Read the model definition and answer for the solid it produces. Units are mm, in the model's axes. Give positions to 0.01 mm unless a question says otherwise; leave off trailing zeros. Loops run counter-clockwise (first coordinate to the right, second up) from the corner with the lowest first, then second, coordinate; pieces in that order, holes last. Notation, with made-up numbers: (79.5, 62.5) - (123.5, 62.5) arc R19 cw to (123.5, 74.5) - close; hole circle Ø5 at (57, 66.25). An arc over 180 degrees is marked (long way). Use a Markdown table: item, result. Add a question column.
Item 1: Consider probe 1 along X at (y, z) = (1.45, 0) (3 decimals); probe 2 along Z at (x, y) = (-0.5, 0.7); probe 3 along Z at (x, y) = (20.5, 1.35). Determine where each line is inside the solid, lowest interval first. Write a range as [from, to].
Item 2: A cutting plane is placed at C-C (y = 1.25). Give the number of separate pieces and of enclosed holes in the cut face, plus the area to 3 significant figures.
Item 3: A cutting plane is placed at A-A (z = 0). Determine the outline of the cut face in (x, y) (3 decimals), plus the area to 3 significant figures.
Item 4: A cutting plane is placed at B-B (x = 0). Determine the outline of the cut face in (y, z) (1 decimal), plus the area to 3 significant figures.
Item 5: Each of these flat-tipped pins is pushed along its axis until it touches: P1, Ø2, axis at x = 21, z = -19.5, coming from the +Y side; P2, Ø1, axis at y = 1, z = -22.5, coming from the -X side; P3, Ø1, axis at y = 1.5, z = -19, coming from the +X side. Where does it stop, or does it pass through?
Item 6: A cutting plane is placed at D-D (x = 20). Determine the outline of the cut face in (y, z).
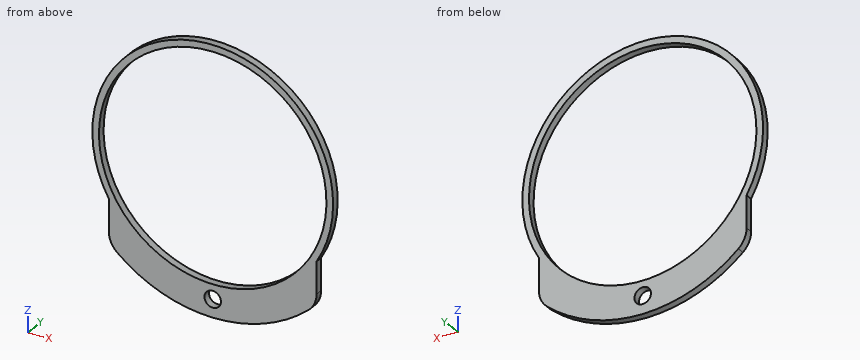
from build123d import *

# Parameters (mm, degrees)
SKETCH1_R           = 32.385
BOSS_EXTRUDE1_DEPTH = 2
FILLET1_R           = 6.35
SKETCH2_R           = 2.2225
CUT_EXTRUDE1_DEPTH  = 52.017498224
SKETCH3_R           = 30.6
CUT_EXTRUDE2_DEPTH  = 52.017498224


with BuildPart() as part:
    # Sketch1 → Boss-Extrude1 (new body)
    with BuildSketch(Plane(origin=(0, 0, 0), x_dir=(1, 0, 0), z_dir=(0, 1, 0))):
        Circle(SKETCH1_R)
        with BuildLine():
            Line((-27.94, 27.737218678), (-27.94, 16.375122137))
            ThreePointArc((-27.94, 16.375122137), (0, 32.385), (27.94, 16.375122137))
            Line((27.94, 16.375122137), (27.94, 27.737218678))
            ThreePointArc((27.94, 27.737218678), (0, 39.37), (-27.94, 27.737218678))
        make_face()
    extrude(amount=BOSS_EXTRUDE1_DEPTH)

    # Fillet1
    fillet1_edges = [part.edges().sort_by_distance(p)[0] for p in [
        (-27.94, 1, -27.737218678),
        (27.94, 1, -27.737218678),
    ]]
    fillet(fillet1_edges, radius=FILLET1_R)

    # Sketch2 → Cut-Extrude1 (cut, through all)
    with BuildSketch(Plane(origin=(0, 2, 0), x_dir=(1, 0, 0), z_dir=(0, 1, 0))):
        with Locations(Location((0, 34.544, 0), (0, 0, 270))):
            Circle(SKETCH2_R)
    extrude(amount=-CUT_EXTRUDE1_DEPTH, mode=Mode.SUBTRACT)

    # Sketch3 → Cut-Extrude2 (cut, through all)
    with BuildSketch(Plane(origin=(0, 2, 0), x_dir=(1, 0, 0), z_dir=(0, 1, 0))):
        with Locations(Location((0, 0, 0), (0, 0, 270))):
            Circle(SKETCH3_R)
    extrude(amount=-CUT_EXTRUDE2_DEPTH, mode=Mode.SUBTRACT)


solid = part.part
Geometry says:
| question | item | result |
|---|---|---|
| 1 | probe 1 | [-32.385, -30.6], [30.6, 32.385] |
| 1 | probe 2 | [-39.37, -36.71], [-32.38, -30.6], [30.6, 32.38] |
| 1 | probe 3 | [-33.61, -22.72], [22.72, 25.07] |
| 2 | separate pieces | 1 |
| 2 | enclosed holes | 2 |
| 2 | area | 785 mm² |
| 3 | outline | (-32.385, 0) - (-30.6, 0) - (-30.6, 2) - (-32.385, 2) - close; (30.6, 0) - (32.385, 0) - (32.385, 2) - (30.6, 2) - close |
| 3 | area | 7.14 mm² |
| 4 | outline | (0, -39.4) - (2, -39.4) - (2, -36.8) - (0, -36.8) - close; (0, -32.3) - (2, -32.3) - (2, -30.6) - (0, -30.6) - close; (0, 30.6) - (2, 30.6) - (2, 32.4) - (0, 32.4) - close |
| 4 | area | 12.2 mm² |
| 5 | P1 | through |
| 5 | P2 | x = -27.94 |
| 5 | P3 | x = 27.94 |
| 6 | outline | (0, -33.91) - (2, -33.91) - (2, -23.16) - (0, -23.16) - close; (0, 23.16) - (2, 23.16) - (2, 25.47) - (0, 25.47) - close |
